Read the model definition and answer for the solid it produces. Units are mm, in the model's axes. A direction names the side the tool comes from. Give positions to 0.01 mm unless a question says otherwise; leave off trailing zeros. Order: outer loops, then holes, each group sorted by start corner. A loop starts at its lowest first (then second) coordinate and runs counter-clockwise, first axis right, second up. Notation, with made-up numbers: (44.5, 67) -> (67.5, 67) arc R23 cw to (67.5, 79) -> close; hole circle Ø2 at (77, 82.5). An arc over 180 degrees is marked (long way). Use one line per item in the form item = value.
```python
from build123d import *

# Parameters (mm, degrees)
SKETCH1_R           = 2.6035
BOSS_EXTRUDE1_DEPTH = 96.04375


with BuildPart() as part:
    # Sketch1 → Boss-Extrude1 (new body, symmetric)
    with BuildSketch(Plane(origin=(0, 0, -450.85), x_dir=(-1, 0, 0), z_dir=(0, 0, -1))):
        with BuildLine():
            Line((12.7, -9.5504), (12.7, -6.3330836))
            ThreePointArc((12.7, -6.3330836), (12.192, -5.8250836), (12.7, -5.3170836))
            Line((12.7, -5.3170836), (12.7, -4.3434))
            ThreePointArc((12.7, -4.3434), (11.5951, -3.2385), (10.4902, -4.3434))
            Line((10.4902, -4.3434), (10.4902, -6.474794456))
            ThreePointArc((10.4902, -6.474794456), (9.863006367, -7.413456061), (8.75577951, -7.193214945))
            Line((8.75577951, -7.193214945), (5.42573597, -3.863171405))
            ThreePointArc((5.42573597, -3.863171405), (4.737482484, -2.833127272), (4.4958, -1.618107374))
            Line((4.4958, -1.618107374), (4.4958, 1.618107374))
            ThreePointArc((4.4958, 1.618107374), (4.737482484, 2.833127272), (5.42573597, 3.863171405))
            Line((5.42573597, 3.863171405), (8.75577951, 7.193214945))
            ThreePointArc((8.75577951, 7.193214945), (9.863006367, 7.413456061), (10.4902, 6.474794456))
            Line((10.4902, 6.474794456), (10.4902, 4.343399971))
            ThreePointArc((10.4902, 4.343399971), (11.5951, 3.238499971), (12.7, 4.343399971))
            Line((12.7, 4.343399971), (12.7, 5.3170836))
            ThreePointArc((12.7, 5.3170836), (12.192, 5.8250836), (12.7, 6.3330836))
            Line((12.7, 6.3330836), (12.7, 9.5504))
            ThreePointArc((12.7, 9.5504), (12.192000006, 10.058323491), (12.699846982, 10.566399977))
            ThreePointArc((12.699846982, 10.566399977), (12.082522516, 12.082522516), (10.566399977, 12.699846982))
            ThreePointArc((10.566399977, 12.699846982), (10.058323491, 12.192000006), (9.5504, 12.7))
            Line((9.5504, 12.7), (6.3330836, 12.7))
            ThreePointArc((6.3330836, 12.7), (5.8250836, 12.192), (5.3170836, 12.7))
            Line((5.3170836, 12.7), (4.3434, 12.7))
            ThreePointArc((4.3434, 12.7), (3.2385, 11.5951), (4.3434, 10.4902))
            Line((4.3434, 10.4902), (6.474794456, 10.4902))
            ThreePointArc((6.474794456, 10.4902), (7.413456061, 9.863006367), (7.193214945, 8.75577951))
            Line((7.193214945, 8.75577951), (3.863171405, 5.42573597))
            ThreePointArc((3.863171405, 5.42573597), (2.833127272, 4.737482484), (1.618107374, 4.4958))
            Line((1.618107374, 4.4958), (-1.618107374, 4.4958))
            ThreePointArc((-1.618107374, 4.4958), (-2.833127272, 4.737482484), (-3.863171405, 5.42573597))
            Line((-3.863171405, 5.42573597), (-7.193214945, 8.75577951))
            ThreePointArc((-7.193214945, 8.75577951), (-7.413456061, 9.863006367), (-6.474794456, 10.4902))
            Line((-6.474794456, 10.4902), (-4.343399971, 10.4902))
            ThreePointArc((-4.343399971, 10.4902), (-3.238499971, 11.5951), (-4.343399971, 12.7))
            Line((-4.343399971, 12.7), (-5.3170836, 12.7))
            ThreePointArc((-5.3170836, 12.7), (-5.8250836, 12.192), (-6.3330836, 12.7))
            Line((-6.3330836, 12.7), (-9.5504, 12.7))
            ThreePointArc((-9.5504, 12.7), (-10.058323491, 12.192000006), (-10.566399977, 12.699846982))
            ThreePointArc((-10.566399977, 12.699846982), (-12.082522516, 12.082522516), (-12.699846982, 10.566399977))
            ThreePointArc((-12.699846982, 10.566399977), (-12.192000006, 10.058323491), (-12.7, 9.5504))
            Line((-12.7, 9.5504), (-12.7, 6.3330836))
            ThreePointArc((-12.7, 6.3330836), (-12.192, 5.8250836), (-12.7, 5.3170836))
            Line((-12.7, 5.3170836), (-12.7, 4.3434))
            ThreePointArc((-12.7, 4.3434), (-11.5951, 3.2385), (-10.4902, 4.3434))
            Line((-10.4902, 4.3434), (-10.4902, 6.474794456))
            ThreePointArc((-10.4902, 6.474794456), (-9.863006367, 7.413456061), (-8.75577951, 7.193214945))
            Line((-8.75577951, 7.193214945), (-5.42573597, 3.863171405))
            ThreePointArc((-5.42573597, 3.863171405), (-4.737482484, 2.833127272), (-4.4958, 1.618107374))
            Line((-4.4958, 1.618107374), (-4.4958, -1.618107374))
            ThreePointArc((-4.4958, -1.618107374), (-4.737482484, -2.833127272), (-5.42573597, -3.863171405))
            Line((-5.42573597, -3.863171405), (-8.75577951, -7.193214945))
            ThreePointArc((-8.75577951, -7.193214945), (-9.863006367, -7.413456061), (-10.4902, -6.474794456))
            Line((-10.4902, -6.474794456), (-10.4902, -4.343399971))
            ThreePointArc((-10.4902, -4.343399971), (-11.5951, -3.238499971), (-12.7, -4.343399971))
            Line((-12.7, -4.343399971), (-12.7, -5.3170836))
            ThreePointArc((-12.7, -5.3170836), (-12.192, -5.8250836), (-12.7, -6.3330836))
            Line((-12.7, -6.3330836), (-12.7, -9.5504))
            ThreePointArc((-12.7, -9.5504), (-12.192000006, -10.058323491), (-12.699846982, -10.566399977))
            ThreePointArc((-12.699846982, -10.566399977), (-12.082522516, -12.082522516), (-10.566399977, -12.699846982))
            ThreePointArc((-10.566399977, -12.699846982), (-10.058323491, -12.192000006), (-9.5504, -12.7))
            Line((-9.5504, -12.7), (-6.3330836, -12.7))
            ThreePointArc((-6.3330836, -12.7), (-5.8250836, -12.192), (-5.3170836, -12.7))
            Line((-5.3170836, -12.7), (-4.3434, -12.7))
            ThreePointArc((-4.3434, -12.7), (-3.2385, -11.5951), (-4.3434, -10.4902))
            Line((-4.3434, -10.4902), (-6.474794456, -10.4902))
            ThreePointArc((-6.474794456, -10.4902), (-7.413456061, -9.863006367), (-7.193214945, -8.75577951))
            Line((-7.193214945, -8.75577951), (-3.863171405, -5.42573597))
            ThreePointArc((-3.863171405, -5.42573597), (-2.833127272, -4.737482484), (-1.618107374, -4.4958))
            Line((-1.618107374, -4.4958), (1.618107374, -4.4958))
            ThreePointArc((1.618107374, -4.4958), (2.833127272, -4.737482484), (3.863171405, -5.42573597))
            Line((3.863171405, -5.42573597), (7.193214945, -8.75577951))
            ThreePointArc((7.193214945, -8.75577951), (7.413456061, -9.863006367), (6.474794456, -10.4902))
            Line((6.474794456, -10.4902), (4.343399971, -10.4902))
            ThreePointArc((4.343399971, -10.4902), (3.238499971, -11.5951), (4.343399971, -12.7))
            Line((4.343399971, -12.7), (5.3170836, -12.7))
            ThreePointArc((5.3170836, -12.7), (5.8250836, -12.192), (6.3330836, -12.7))
            Line((6.3330836, -12.7), (9.5504, -12.7))
            ThreePointArc((9.5504, -12.7), (10.058323491, -12.192000006), (10.566399977, -12.699846982))
            ThreePointArc((10.566399977, -12.699846982), (12.082522516, -12.082522516), (12.699846982, -10.566399977))
            ThreePointArc((12.699846982, -10.566399977), (12.192000006, -10.058323491), (12.7, -9.5504))
        make_face()
        Circle(SKETCH1_R, mode=Mode.SUBTRACT)
    extrude(amount=BOSS_EXTRUDE1_DEPTH, both=True)


solid = part.part
```
Item 1: The part is cut by section A-A on x = 0. Give the vertices of the cut face in (y, z), and give its area (3 significant figures).
Checks:
outline = (-4.5, -546.89) -> (-2.6, -546.89) -> (-2.6, -354.81) -> (-4.5, -354.81) -> close; (2.6, -546.89) -> (4.5, -546.89) -> (4.5, -354.81) -> (2.6, -354.81) -> close
area = 727 mm²
Item 2: Given pin 1 Ø1.6 at (x, z) = (0, -455.5) entering from +Y; pin 2 Ø3.5 at (y, z) = (-0.5, -476.5) entering from +X; pin 3 Ø1.6 at (y, z) = (0.5, -492.5) entering from -X, each flat-ended and moving along its own axis, determine where each tip first touches the part or whether it passes through.
Checks:
pin_1 = 4.5
pin_2 = 4.56
pin_3 = -4.5
Item 3: Which of the six approach directions +Z, -Z, +X, -X, +Y, -Y give full straight-line access (tool end or side, diameter ignored) to faces 4 (the flat face through (0, -4.496, -452)), 5 (the flat face through (7.11, 5.55, -452.19)), 6 (the flat face through (-4.496, 0, -452)), 7 (the flat face through (-8, -12.7, -452)), 8 (the flat face through (4.496, 0, -452))?
Checks:
face_4 = +Z, -Z, -Y
face_5 = +Z, -Z
face_6 = +Z, -Z, -X
face_7 = +Z, -Z, +X, -X, -Y
face_8 = +Z, -Z, +X
Item 4: Determine the mould class of faces 1 (the flat face through (-5.505, -7.067, -452.195)), 2 (the flat face through (8, 12.7, -452)), 3 (the flat face through (12.7, -8, -452)) for opening direction X: +X half, -X half, draft (parallel to the pull), parting line (faces both ways), or undercut.
Checks:
face_1 = undercut
face_2 = draft
face_3 = +X half
Item 5: Straight lines are drawn through the part: L1, parallel to Y at x = 0, z = -409.5; L2, parallel to X at y = -4.25, z = -390; L3, parallel to Y at x = 6.75, z = -492.5. For each, find the intervals that lie inside material, in ascending order. Write a range as from..to.
Checks:
L1 = -4.5..-2.6, 2.6..4.5
L2 = -12.7..-10.49, -5.81..5.81, 10.49..12.7
L3 = -12.7..-10.45, -8.31..-5.19, 5.19..8.31, 10.45..12.7
